Geometry: final body of the model. Coordinates: model frame, mm. Face numbers are marked on the shaded views. A direction names the side the tool comes from. Round coordinates to 2 decimals unless told otherwise and drop trailing zeros. Loops run counter-clockwise (first coordinate to the right, second up) from the corner with the lowest first, then second, coordinate; pieces in that order, holes last. Notation, with made-up numbers: (25, -28.75) - (75, -28.75) arc R12 cw to (75, -19.75) - close; hole circle Ø1 at (0, 81). An arc over 180 degrees is marked (long way). Return JSON: item names as keys, results as strings. Group by question number.
1. Material intervals for probe 1 along Z at (x, y) = (-25, 7); probe 2 along X at (y, z) = (15.5, -55); probe 3 along Z at (x, y) = (4, -6), sorted ascending.
2. Section A-A on y = 16.5. Return loops of the section in (x, z), and give its area (3 significant figures).
3. Section C-C on z = -16. Return loops of the section in (x, y).
4. First-contact query: pin 1 Ø7.5 at (x, z) = (25, 55) entering from -Y; pin 2 Ø1.5 at (x, z) = (-36, 3.5) entering from +Y; pin 3 Ø19.5 at (x, z) = (1, -14.5) entering from -Y; pin 4 Ø9 at (x, y) = (-7, -4) entering from -Z. Flat tips, straight axial feed; report the tip coordinate or a pass-through.
5. Set-up query: the marked faces 1, 2 and 3. Return all of +Z, -Z, +X, -X, +Y, -Y with unobstructed straight access to the full face (end or side cutting, diameter ignored); none if empty.
6. Section D-D on x = -26.5. Count the separate pieces of the cut face and the enclosed holes in it, and give its area (3 significant figures).
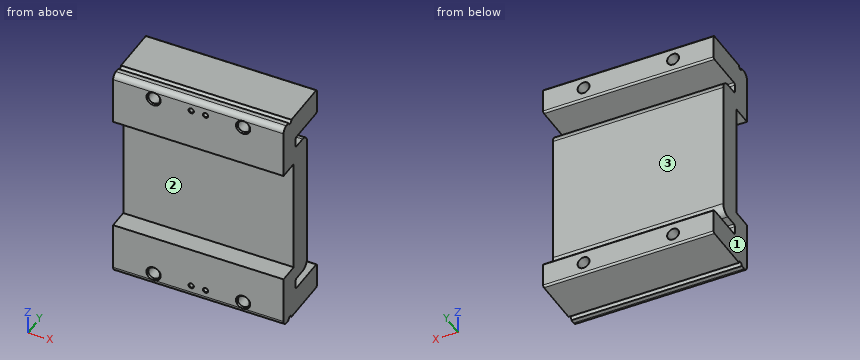
Autodesk Inventor part; units mm, degrees
ref_plane "slider_spacer_sensor_dog_XY" through (0, -11, 55) normal (0, 1, 0) x (1, 0, 0)
ref_plane "slider_spacer_sensor_dog_YZ" through (0, -11, 55) normal (1, 0, 0) x (0, 0, -1)
ref_plane "slider_spacer_sensor_dog_ZX" through (0, -11, 55) normal (0, 0, -1) x (0, 1, 0)
sketch "Sketch_1" plane through (0, 0, 0) normal (1, 0, 0) x (0, 1, 0)
  line L0 (24, 62) -> (-2.5, 62)
  arc A0 (-5.5, 62) -> (-2.5, 62) centre (-4, 62) ccw
  line L1 (-5.5, 62) -> (-8, 62)
  arc A1 (-8, 62) -> (-11, 59) centre (-8, 59) ccw
  line L2 (-11, 59) -> (-11, 32.5)
  line L3 (-11, 32.5) -> (0, 32.5)
  line L4 (0, 32.5) -> (0, -32.5)
  line L5 (0, -32.5) -> (-11, -32.5)
  line L6 (-11, -32.5) -> (-11, -59)
  arc A2 (-11, -59) -> (-8, -62) centre (-8, -59) ccw
  line L7 (-8, -62) -> (-5.5, -62)
  arc A3 (-2.5, -62) -> (-5.5, -62) centre (-4, -62) ccw
  line L8 (-2.5, -62) -> (24, -62)
  arc A4 (24, -62) -> (25, -61) centre (24, -61) ccw
  line L9 (25, -61) -> (25, -48.5)
  arc A5 (25, -48.5) -> (24, -47.5) centre (24, -48.5) ccw
  line L10 (24, -47.5) -> (3, -47.5)
  arc A6 (2, -46.5) -> (3, -47.5) centre (3, -46.5) ccw
  line L11 (2, -46.5) -> (2, -42.5)
  arc A7 (3, -41.5) -> (2, -42.5) centre (3, -42.5) ccw
  line L12 (3, -41.5) -> (9.5, -41.5)
  arc A8 (9.5, -41.5) -> (14.5, -36.5) centre (9.5, -36.5) ccw
  line L13 (14.5, -36.5) -> (14.5, 36.5)
  arc A9 (14.5, 36.5) -> (9.5, 41.5) centre (9.5, 36.5) ccw
  line L14 (9.5, 41.5) -> (3, 41.5)
  arc A10 (2, 42.5) -> (3, 41.5) centre (3, 42.5) ccw
  line L15 (2, 42.5) -> (2, 46.5)
  arc A11 (3, 47.5) -> (2, 46.5) centre (3, 46.5) ccw
  line L16 (3, 47.5) -> (24, 47.5)
  arc A12 (24, 47.5) -> (25, 48.5) centre (24, 48.5) ccw
  line L17 (25, 48.5) -> (25, 61)
  arc A13 (25, 61) -> (24, 62) centre (24, 61) ccw
extrude "Extrusion1" add sketch "Sketch_1" along normal mid plane 95.2
sketch "Sketch2" plane through (-47.6, -11, 59) normal (0, -1, 0) x (1, 0, 0)
  point P0 (22.6, -4)
hole "Drilling 1" at (-25, -11, 55) direction (0, 1, 0) diameter 6.647 depth 36 countersink diameter 8 countersink angle 90
pattern_linear "Rectangular Pattern1" count 2 spacing 50 along (1, 0, 0) count 2 spacing 110 along (0, 0, -1) of "Drilling 1"
sketch "Sketch3" plane through (-47.6, -11, 32.5) normal (0, -1, 0) x (1, 0, 0)
  point P0 (43.6, 22.5)
hole "Drilling 2" at (-4, -11, 55) direction (0, 1, 0) diameter 2.459 depth 7 tip angle 140 countersink diameter 3 countersink angle 90
pattern_linear "Rectangular Pattern2" count 2 spacing 8 along (1, 0, 0) count 2 spacing 110 along (0, 0, -1) of "Drilling 2"
ref_plane "slider_spacer_sensor_dog_XY" through (0, -11, 55) normal (0, 1, 0) x (1, 0, 0)
ref_plane "slider_spacer_sensor_dog_YZ" through (0, -11, 55) normal (1, 0, 0) x (0, 0, -1)
ref_plane "slider_spacer_sensor_dog_ZX" through (0, -11, 55) normal (0, 0, -1) x (0, 1, 0)
ref_plane "slider_spacer_slider_XY" through (0, 0, 0) normal (0, 1, 0) x (1, 0, 0)
ref_plane "slider_spacer_slider_YZ" through (0, 0, 0) normal (1, 0, 0) x (0, 0, -1)
ref_plane "slider_spacer_slider_ZX" through (0, 0, 0) normal (0, 0, -1) x (0, 1, 0)
properties part number "KR55-A-Slider Spacer"
Taken from the geometry:
{
 "1": {"probe 1": "-62 to -58.32, -51.68 to -47.5, -41.5 to 41.5, 47.5 to 51.68, 58.32 to 62", "probe 2": "-47.6 to -28.32, -21.68 to 21.68, 28.32 to 47.6", "probe 3": "-62 to -56.23, -53.77 to -32.5, 32.5 to 53.77, 56.23 to 62"},
 "2": {"outline": "(-47.6, -62) - (47.6, -62) - (47.6, -47.5) - (-47.6, -47.5) - close; (-47.6, 47.5) - (47.6, 47.5) - (47.6, 62) - (-47.6, 62) - close; hole circle Ø6.65 at (-25, -55); hole circle Ø6.65 at (-25, 55); hole circle Ø6.65 at (25, -55); hole circle Ø6.65 at (25, 55)", "area": "2,620 mm2"},
 "3": {"outline": "(-47.6, 0) - (47.6, 0) - (47.6, 14.5) - (-47.6, 14.5) - close"},
 "4": {"pin 1": "y = -10.75", "pin 2": "y = 14.5", "pin 3": "y = 0", "pin 4": "z = -62"},
 "5": {"face 1": "+Z, -Z, -X, +Y, -Y", "face 2": "+X, -X, -Y", "face 3": "+X, -X, +Y"},
 "6": {"separate pieces": "3", "enclosed holes": "0", "area": "2,150 mm2"}
}
